CAD build for the part. Positions are in the model's coordinates, mm. Face numbers are marked on the shaded views. A direction names the side the tool comes from. Coordinates: 2 decimals unless noted, no trailing zeros. Loops run counter-clockwise (first coordinate to the right, second up) from the corner with the lowest first, then second, coordinate; pieces in that order, holes last.
1) Wall check: line 1 along Z through (x, y) = (-2.5, -43); line 2 along X through (y, z) = (-55, 23.5); line 3 along Y through (x, z) = (-9, 56.5). Give the ranges that are in metal, low to high.
2) Pin check, flat tips, straight feed: pin 1 Ø19 at (x, y) = (28, -39) entering from +Z; pin 2 Ø4 at (x, z) = (33.5, 30) entering from -Y. Stop position of each tip, or through.
3) Saw through at B-B, the plane z = 17.5. Write the cut outline in (x, y), and give its area (3 significant figures).
4) Which spindle directions (+Z, -Z, +X, -X, +Y, -Y) get a long thin tool onto all of the face, cutting with end or side? Do the marked faces 1 and 2. Say none if no direction does.
5) Saw through at A-A, the plane y = -56.5. Write the cut outline in (x, z), and give its area (3 significant figures).
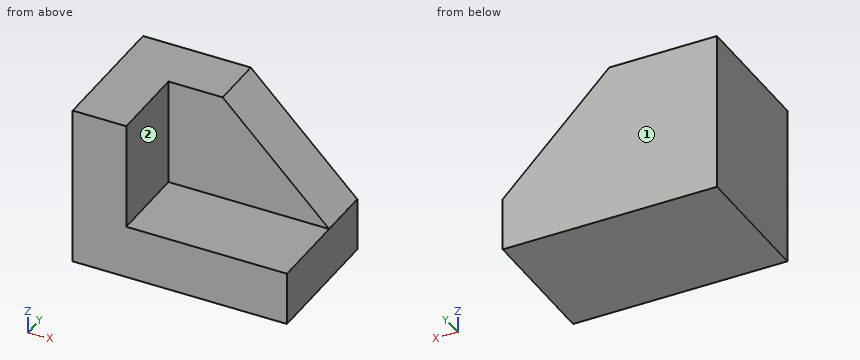
```python
from build123d import *

# Parameters (mm, degrees)
F0_W     = 101.6
F0_H     = 25.4
F1_DEPTH = 63.5
F2_W     = 25.4
F2_H     = 63.5
F3_DEPTH = 50.8
F4_W     = 25.709516
F4_H     = 25.4
F5_DEPTH = 50.8
F7_DEPTH = 25.4


with BuildPart() as f1:
    # F0 (on Front) → F1 (new body)
    with BuildSketch(Plane.XZ):
        with Locations((-0.309516, 3.400826)):
            Rectangle(F0_W, F0_H)
    extrude(amount=F1_DEPTH)

    # F2 (on face) → F3 (join)
    with BuildSketch(Plane.XY.offset(16.100826)):
        with Locations((-38.409516, -31.75)):
            Rectangle(F2_W, F2_H)
    extrude(amount=F3_DEPTH)

    # F4 (on face) → F5 (join)
    with BuildSketch(Plane.XY.offset(16.100826)):
        with Locations((-12.854758, -12.7)):
            Rectangle(F4_W, F4_H)
    extrude(amount=F5_DEPTH)

    # F6 (on face) → F7 (join)
    with BuildSketch(Plane.XZ.offset(25.4)):
        Polygon((50.451178, 16.100826), (0, 66.900826), (0, 16.100826), align=None)
    extrude(amount=-F7_DEPTH)


solid = f1.part
```
Data:
1. line 1: z = -9.3 to 16.1
1. line 2: x = -51.11 to -25.71
1. line 3: y = -25.4 to 0
2. pin 1: stops at z = 16.1
2. pin 2: stops at y = -25.4
3. outline: (-51.11, -63.5) - (-25.71, -63.5) - (-25.71, -25.4) - (49.06, -25.4) - (49.06, 0) - (-51.11, 0) - close
3. area: 3,510 mm2
4. face 1: +Z, -Z, +X, -X, +Y
4. face 2: +Z, +X, -Y
5. outline: (-51.11, -9.3) - (50.49, -9.3) - (50.49, 16.1) - (-25.71, 16.1) - (-25.71, 66.9) - (-51.11, 66.9) - close
5. area: 3,870 mm2
